Could you check a few things on this model? Use its own coordinates, in mm. Round coordinates to 2 decimals unless told otherwise and drop trailing zeros. Order: outer loops, then holes, each group sorted by start corner. A loop starts at its lowest first (then second) coordinate and runs counter-clockwise, first axis right, second up. Notation, with made-up numbers: (64, 69.5) -> (111, 69.5) arc R22 ccw to (111, 94.5) -> close; hole circle Ø9 at (14, -26). An arc over 180 degrees is marked (long way). One line per question, with ' | ' between items.
```python
from build123d import *

# Parameters (mm, degrees)
F0_W     = 200
F0_H     = 21
F1_DEPTH = 21
F2_W     = 11
F2_H     = 11
F3_DEPTH = 200


with BuildPart() as f1:
    # F0 (on Front) → F1 (new body)
    with BuildSketch(Plane.XZ):
        with Locations((-100, 10.5)):
            Rectangle(F0_W, F0_H)
    extrude(amount=F1_DEPTH)

    # F2 (on Right) → F3 (cut)
    with BuildSketch(Plane.YZ):
        with Locations((-10.5, 10.5)):
            Rectangle(F2_W, F2_H)
    extrude(amount=-F3_DEPTH, mode=Mode.SUBTRACT)


solid = f1.part
```
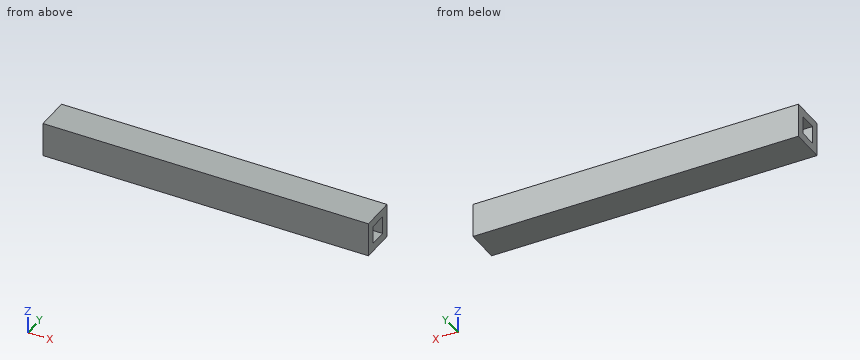
1. I want a section at B-B on z = 8. List the corners of the cut face in (x, y) for me.
From the geometry:
outline: (-200, -21) -> (0, -21) -> (0, -16) -> (-200, -16) -> close; (-200, -5) -> (0, -5) -> (0, 0) -> (-200, 0) -> close
2. I want a section at A-A on y = -12.25. List the corners of the cut face in (x, z) for me.
From the geometry:
outline: (-200, 0) -> (0, 0) -> (0, 5) -> (-200, 5) -> close; (-200, 16) -> (0, 16) -> (0, 21) -> (-200, 21) -> close
3. I need wall thicknesses on probe 1 along Y at (x, z) = (-129.5, 6.25); probe 2 along Z at (x, y) = (-36.5, -14.5). Which ranges of each line are inside material? Lowest first, please.
From the geometry:
probe 1: y = -21 to -16, -5 to 0 | probe 2: z = 0 to 5, 16 to 21
4. I want a section at C-C on x = -166. List the corners of the cut face in (y, z) for me.
From the geometry:
outline: (-21, 0) -> (0, 0) -> (0, 21) -> (-21, 21) -> close; hole (-16, 5) -> (-5, 5) -> (-5, 16) -> (-16, 16) -> close
